Model file for the job. Use its own axes, mm. Round coordinates to 2 decimals unless told otherwise and drop trailing zeros. Order: outer loops, then holes, each group sorted by start corner. A loop starts at its lowest first (then second) coordinate and runs counter-clockwise, first axis right, second up. Notation, with made-up numbers: (0.25, 0.5) - (7.25, 0.5) arc R24 ccw to (7.25, 15.5) - close; hole circle Ø6 at (54.25, 77). An arc over 180 degrees is marked (long way). Write item = value, one per line.
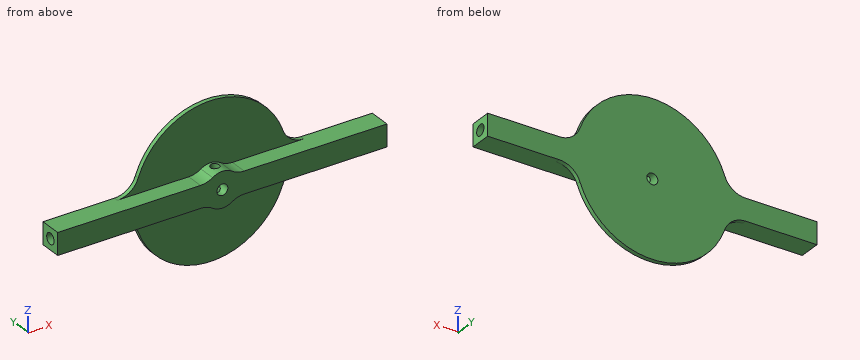
```python
from build123d import *

# Parameters (mm, degrees)
F0_R          = 2.5
F1_DEPTH      = 10
F2_R          = 35
F2_R_2        = 2.5
F3_DEPTH      = 2
F4_R          = 2.5
F5_DEPTH      = 25
F6_R          = 2
F7_DEPTH      = 35.001
F7_DEPTH_BACK = 35.001
F8_R          = 10


# Not quite as in the source:
# - a pattern or mirror of a feature is missing from the dataset's text; its kind, count and spacing are read off the source's solid


with BuildPart() as f1:
    # F0 (on Front) → F1 (new body)
    with BuildSketch(Plane.XZ):
        with BuildLine():
            Line((75, 5), (6.2449979984, 5))
            ThreePointArc((6.2449979984, 5), (0, 8), (-6.2449979984, 5))
            Line((-6.2449979984, 5), (-75, 5))
            Line((-75, 5), (-75, -5))
            Line((-75, -5), (-6.2449979984, -5))
            ThreePointArc((-6.2449979984, -5), (0, -8), (6.2449979984, -5))
            Line((6.2449979984, -5), (75, -5))
            Line((75, -5), (75, 5))
        make_face()
        Circle(F0_R, mode=Mode.SUBTRACT)
    extrude(amount=F1_DEPTH)

    # F2 (on face) → F3 (join)
    with BuildSketch(Plane(origin=(0, 0, 0), x_dir=(-1, 0, 0), z_dir=(0, 1, 0))):
        Circle(F2_R)
        Circle(F2_R_2, mode=Mode.SUBTRACT)
    extrude(amount=-F3_DEPTH)

    # F4 (on face) → F5 (cut)
    with BuildSketch(Plane(origin=(-75, 0, 0), x_dir=(0, -1, 0), z_dir=(-1, 0, 0))):
        with Locations((5, 0)):
            Circle(F4_R)
    f5 = extrude(amount=-F5_DEPTH, mode=Mode.SUBTRACT)

    # F5_copies: F5 across plane
    add(f5.mirror(Plane(origin=(0, 0, 0), x_dir=(0, 0, 1), z_dir=(1, 0, 0))), mode=Mode.SUBTRACT)

    # F6 (on Top) → F7 (cut, two sides)
    with BuildSketch(Plane.XY) as f7_sk:
        with Locations((0, -5)):
            Circle(F6_R)
    extrude(amount=-F7_DEPTH, mode=Mode.SUBTRACT)
    extrude(f7_sk.sketch, amount=F7_DEPTH_BACK, mode=Mode.SUBTRACT)

    # F8
    f8_edges = [f1.edges().sort_by_distance(p)[0] for p in [
        (-6.244998, -6, 5),
        (6.244998, -6, 5),
        (6.244998, -6, -5),
        (-6.244998, -6, -5),
        (34.641016, -1, 5),
        (34.641016, -1, -5),
        (-34.641016, -1, -5),
        (-34.641016, -1, 5),
    ]]
    fillet(f8_edges, radius=F8_R)


solid = f1.part
```
1) Cut at C-C (y = -5). Write the cut outline in (x, z), and give its area (3 significant figures).
Conclusion:
outline = (-75, -5) - (-9.95, -5) arc R10 cw to (-4.42, -6.67) arc R8 ccw to (-2, -7.75) - (-2, -1.5) arc R2.5 cw to (-2, 1.5) - (-2, 7.75) arc R8 ccw to (-4.42, 6.67) arc R10 cw to (-9.95, 5) - (-75, 5) - (-75, 2.5) - (-50, 2.5) - (-50, -2.5) - (-75, -2.5) - close; (2, -7.75) arc R8 ccw to (4.42, -6.67) arc R10 cw to (9.95, -5) - (75, -5) - (75, -2.5) - (50, -2.5) - (50, 2.5) - (75, 2.5) - (75, 5) - (9.95, 5) arc R10 cw to (4.42, 6.67) arc R8 ccw to (2, 7.75) - (2, 1.5) arc R2.5 cw to (2, -1.5) - close
area = 1,240 mm^2
2) Cut at A-A (z = 0). Write the cut outline in (x, y).
Conclusion:
outline = (-75, -10) - (-2.5, -10) - (-2.5, 0) - (-75, 0) - (-75, -2.5) - (-50, -2.5) - (-50, -7.5) - (-75, -7.5) - close; (2.5, -10) - (75, -10) - (75, -7.5) - (50, -7.5) - (50, -2.5) - (75, -2.5) - (75, 0) - (2.5, 0) - close
3) Wall check: line 1 along Z through (x, y) = (55.75, -5); line 2 along Z through (x, y) = (-39, -2.5); line 3 along Y through (x, z) = (-6, 7). Give the ranges that are in metal, low to high.
Conclusion:
line_1 = -5 to -2.5, 2.5 to 5
line_2 = -5 to 5
line_3 = -2 to 0
4) Flat gauge pins, fed straight in: pin 1 Ø3 at (x, y) = (-5.5, -8) entering from -Z; pin 2 Ø4.5 at (x, y) = (0, -5) entering from +Z; pin 3 Ø9 at (x, z) = (-20, 22.5) entering from -Y; pin 4 Ø3 at (x, y) = (0, -5) entering from -Z. Where does each tip first touch, or does it go through?
Conclusion:
pin_1 = -6.93
pin_2 = 8
pin_3 = -2
pin_4 = through
5) Cut at B-B (x = 0). Write the cut outline in (y, z).
Conclusion:
outline = (-10, -8) - (-7, -8) - (-7, -2.5) - (-10, -2.5) - close; (-10, 2.5) - (-7, 2.5) - (-7, 8) - (-10, 8) - close; (-3, -8) - (-2, -8) - (-2, -35) - (0, -35) - (0, -2.5) - (-3, -2.5) - close; (-3, 2.5) - (0, 2.5) - (0, 35) - (-2, 35) - (-2, 8) - (-3, 8) - close
6) Cut at D-D (x = 38.5). Write the cut outline in (y, z).
Conclusion:
outline = (-10, -5) - (-2, -5) - (-2, -5.8) - (0, -5.8) - (0, 5.8) - (-2, 5.8) - (-2, 5) - (-10, 5) - close
